from build123d import *

# Parameters (mm, degrees)
SKETCH1_R                      = 45
BOSS_EXTRUDE1_DEPTH            = 5
F_6_1_6_1_DIAMETER_HOLE1_D     = 6.1
F_6_1_6_1_DIAMETER_HOLE1_DEPTH = 10
F_6_1_6_1_DIAMETER_HOLE1_TIP   = 1.832624888


with BuildPart() as part:
    # Sketch1 → Boss-Extrude1 (new body)
    with BuildSketch(Plane.XY):
        Circle(SKETCH1_R)
    extrude(amount=BOSS_EXTRUDE1_DEPTH)

    # Ø6.1 (6.1) Diameter Hole1
    with Locations(Plane.XY.offset(5)):
        with Locations((-35, 0), (-30.310889132, 17.5), (-17.5, 30.310889132), (0, 35), (17.5, 30.310889132), (30.310889132, 17.5), (35, 0), (30.310889132, -17.5), (17.5, -30.310889132), (0, -35), (-17.5, -30.310889132), (-30.310889132, -17.5)):
            Hole(F_6_1_6_1_DIAMETER_HOLE1_D / 2, depth=F_6_1_6_1_DIAMETER_HOLE1_DEPTH)
            with Locations((0, 0, -(F_6_1_6_1_DIAMETER_HOLE1_DEPTH + F_6_1_6_1_DIAMETER_HOLE1_TIP / 2))):  # 118° drill point
                Cone(0, F_6_1_6_1_DIAMETER_HOLE1_D / 2, F_6_1_6_1_DIAMETER_HOLE1_TIP, mode=Mode.SUBTRACT)


solid = part.part
For this review, take the finished solid that the model builds, in its own axes (mm). Give positions to 0.01 mm unless a question says otherwise; leave off trailing zeros. Loops run counter-clockwise (first coordinate to the right, second up) from the corner with the lowest first, then second, coordinate; pieces in that order, holes last.
Item 1: Draft analysis for pull direction X (two halves, no side actions). For faces 1 (the flat face through (-1, 1, 5)), 2 (the cylindrical face through (20.765, -39.923, 2.465)), 3 (the cylindrical face through (-17.103, 33.335, 2.465)), state which applies: +X half, -X half, draft (parallel to the pull), parting line (faces both ways), or undercut.
Item 2: Take a section at C-C, the plane z = 4.15. Give the number of separate pieces and of enclosed holes in the cut face, and give its area (3 significant figures).
Item 3: Insertion check: pin 1 (2 mm diameter, centred on x = 26, z = 2, fed in from -Y). The pin has a flat end and moves straight along its axis. Give the tip position at first contact, or say it passes through.
Item 4: Take a section at D-D, the plane x = -35. State the section outline as (y, z) points.
Item 5: For line 1 along Y through (x, z) = (-1.5, 0.9) (3 decimals); line 2 along X through (y, z) = (17, 2.2); line 3 along X through (y, z) = (30, 3.4), list the stretches that pass through material, from the lowest coordinate up.
Item 6: Take a section at A-A, the plane x = 0. State the section outline as (y, z) points, and give its area (3 significant figures).
Calculated:
1. face 1: draft
1. face 2: parting line
1. face 3: undercut
2. separate pieces: 1
2. enclosed holes: 12
2. area: 6,010 mm2
3. pin 1: stops at y = -37.42
4. outline: (-28.28, 0) - (-3.05, 0) - (-3.05, 5) - (-28.28, 5) - close; (3.05, 0) - (28.28, 0) - (28.28, 5) - (3.05, 5) - close
5. line 1: y = -44.975 to -37.656, -32.344 to 32.344, 37.656 to 44.975
5. line 2: x = -41.67 to -33.32, -27.3 to 27.3, 33.32 to 41.67
5. line 3: x = -33.54 to -20.53, -14.47 to 14.47, 20.53 to 33.54
6. outline: (-45, 0) - (-38.05, 0) - (-38.05, 5) - (-45, 5) - close; (-31.95, 0) - (31.95, 0) - (31.95, 5) - (-31.95, 5) - close; (38.05, 0) - (45, 0) - (45, 5) - (38.05, 5) - close
6. area: 389 mm2
